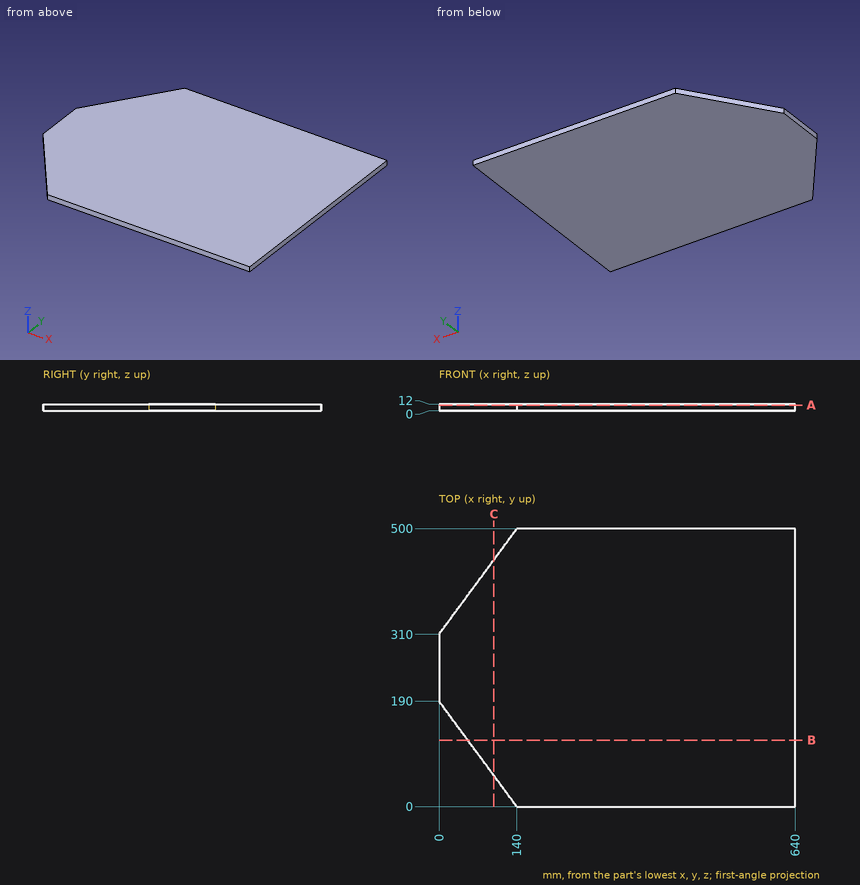
Verification items for this drawing (mm, ordinates from the low corner). Coordinates: 2 decimals unless noted, no trailing zeros. Order: outer loops, then holes, each group sorted by start corner. A loop starts at its lowest first (then second) coordinate and runs counter-clockwise, first axis right, second up. Notation, with made-up numbers: M 78.5,-34.75 L 89.5,-34.75 A27 cw 89.5,-9.75 Z; hole C 69,69 d7. An arc over 180 degrees is marked long. Use CSV: the item, a comma, the result in double quotes.
Item 1: Cross-section at A-A on z = 10. Record the cut outline in (x, y), then the cut area to 3 significant figures.
Returned:
outline,"M 0,190 L 140,0 L 640,0 L 640,500 L 140,500 L 0,310 Z"
area,"293,000 mm2"
Item 2: Thickness scan on line 1 along X through (y, z) = (130.5, 9); line 2 along X through (y, z) = (434.5, 11.25); line 3 along Y through (x, z) = (50.5, 6). Record the ranges inside material, lowest first.
Returned:
line 1,"x = 43.84 to 640"
line 2,"x = 91.74 to 640"
line 3,"y = 121.46 to 378.54"
Item 3: Cross-section at B-B on y = 120. Record the cut outline in (x, z), then the cut area to 3 significant figures.
Returned:
outline,"M 51.58,0 L 640,0 L 640,12 L 51.58,12 Z"
area,"7,060 mm2"
Item 4: Cross-section at C-C on x = 98.5. Record the cut outline in (y, z).
Returned:
outline,"M 56.32,0 L 443.68,0 L 443.68,12 L 56.32,12 Z"
